Geometry check sheet. Reference: the model listing, model coordinates, mm. Coordinates: 2 decimals unless noted, no trailing zeros. Loops run counter-clockwise (first coordinate to the right, second up) from the corner with the lowest first, then second, coordinate; pieces in that order, holes last. Notation, with made-up numbers: M 69,-14.5 L 121,-14.5 A17 ccw 121,13.5 Z; hole C -12.5,87 d9. An arc over 180 degrees is marked long. Use CSV: the item, a comma, the result in double quotes.
```python
from build123d import *

# Parameters (mm, degrees)
F0_R            = 50.8
F2_DEPTH        = 6.35
F1_R            = 11.049
F3_DEPTH        = 10.414
F5_R            = 11.049
F6_DEPTH        = 6.35
F6_COPIES_COUNT = 6


# Not quite as in the source:
# - a pattern or mirror of a feature is missing from the dataset's text; its kind, count and spacing are read off the source's solid
# - a feature names something its author has since deleted; it is built from what else it names


with BuildPart() as f2:
    # F0 (on Front) → F2 (new body)
    with BuildSketch(Plane.XZ):
        Circle(F0_R)
    extrude(amount=F2_DEPTH)

    # F1 (on Front) → F3 (cut)
    with BuildSketch(Plane.XZ):
        Circle(F1_R)
    extrude(amount=F3_DEPTH, mode=Mode.SUBTRACT)

    # F5 (on Front) → F6 (cut)
    with BuildSketch(Plane.XZ):
        with Locations((0, -34.7183458507)):
            Circle(F5_R)
    f6 = extrude(amount=F6_DEPTH, mode=Mode.SUBTRACT)

    # F6_copies: F6 ×6 about axis
    f6_copies_axis = Axis((0, 0, 0), (0, 1, 0))
    for i in range(1, F6_COPIES_COUNT):
        add(f6.rotate(f6_copies_axis, i * 360 / F6_COPIES_COUNT), mode=Mode.SUBTRACT)


solid = f2.part
```
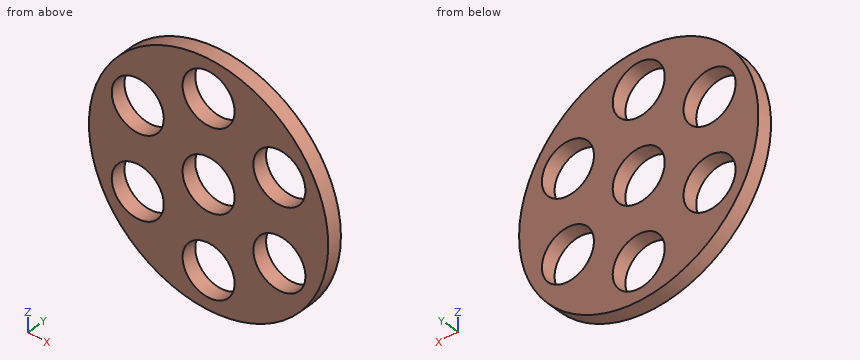
1. Section check A-A, the plane x = 0. Record the cut outline in (y, z).
The answers:
outline,"M -6.35,-50.8 L 0,-50.8 L 0,-45.77 L -6.35,-45.77 Z; M -6.35,-23.67 L 0,-23.67 L 0,-11.05 L -6.35,-11.05 Z; M -6.35,11.05 L 0,11.05 L 0,23.67 L -6.35,23.67 Z; M -6.35,45.77 L 0,45.77 L 0,50.8 L -6.35,50.8 Z"
2. Thickness scan on line 1 (Z direction, x = 0, y = -3.25); line 2 (Z direction, x = 33.5, y = -1.5); line 3 (Z direction, x = 37.5, y = -5.5). Record the ranges inside material, lowest first. Write a range as [from, to].
The answers:
line 1,"[-50.8, -45.77], [-23.67, -11.05], [11.05, 23.67], [45.77, 50.8]"
line 2,"[-38.19, -27.86], [-6.86, 6.86], [27.86, 38.19]"
line 3,"[-34.27, -25.53], [-9.18, 9.18], [25.53, 34.27]"
3. Section check C-C, the plane x = 29. Record the cut outline in (y, z).
The answers:
outline,"M -6.35,-41.71 L 0,-41.71 L 0,-28.36 L -6.35,-28.36 Z; M -6.35,-6.36 L 0,-6.36 L 0,6.36 L -6.35,6.36 Z; M -6.35,28.36 L 0,28.36 L 0,41.71 L -6.35,41.71 Z"
4. Section check D-D, the plane z = -17. Record the cut outline in (x, y), plus the area to 3 significant figures.
The answers:
outline,"M -47.87,-6.35 L -41.11,-6.35 L -41.11,0 L -47.87,0 Z; M -19.02,-6.35 L 19.02,-6.35 L 19.02,0 L -19.02,0 Z; M 41.11,-6.35 L 47.87,-6.35 L 47.87,0 L 41.11,0 Z"
area,"327 mm^2"
5. Gauge pin test, flat ends, axial feed: P1, Ø17.5, axis at x = 0, z = -34.72, coming from the -Y side; P2, Ø3, axis at x = -2, y = -1, coming from the +Z side; P3, Ø6, axis at x = 30.5, z = -34.5, coming from the +Y side; P4, Ø1.5, axis at y = -2, z = 23, coming from the -X side. Record the tip position at first contact, or that the pin passes through.
The answers:
P1,"through"
P2,"z = 50.8"
P3,"y = 0"
P4,"x = -45.67"
6. Section check B-B, the plane z = 0. Record the cut outline in (x, y), plus the area to 3 significant figures.
The answers:
outline,"M -50.8,-6.35 L -11.05,-6.35 L -11.05,0 L -50.8,0 Z; M 11.05,-6.35 L 50.8,-6.35 L 50.8,0 L 11.05,0 Z"
area,"505 mm^2"
